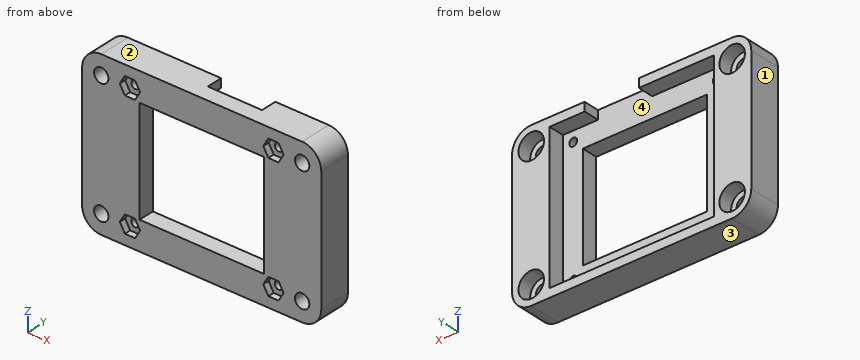
from build123d import *

# Parameters (mm, degrees)
SKETCH_1_W                   = 75
SKETCH_1_H                   = 51
EXTRUDE_1_DEPTH              = 10
SKETCH_2_W                   = 51.5
SKETCH_2_H                   = 45.5
CUT_EXTRUDE_1_DEPTH          = 5
SKETCH_3_R                   = 1.25
CUT_EXTRUDE_2_DEPTH          = 5
CUT_EXTRUDE_3_REACH          = 7
SKETCH_4_W                   = 39
SKETCH_4_H                   = 33
FILLET_1_R                   = 6
CUT_EXTRUDE_4_DEPTH          = 2
HOLE_WIZARD_M4_1_D           = 4.5
HOLE_WIZARD_M4_1_CBORE_D     = 8
HOLE_WIZARD_M4_1_CBORE_DEPTH = 4.4
SKETCH_7_W                   = 17
SKETCH_7_H                   = 2.75
CUT_EXTRUDE_5_DEPTH          = 5


with BuildPart() as part:
    # 草图1 → 凸台-拉伸1 (new body)
    with BuildSketch(Plane(origin=(0, 0, 0), x_dir=(1, 0, 0), z_dir=(0, 1, 0))):
        Rectangle(SKETCH_1_W, SKETCH_1_H)
    extrude(amount=EXTRUDE_1_DEPTH)

    # 草图2 → 切除-拉伸1 (cut)
    with BuildSketch(Plane(origin=(0, 10, 0), x_dir=(1, 0, 0), z_dir=(0, 1, 0))):
        Rectangle(SKETCH_2_W, SKETCH_2_H)
    extrude(amount=-CUT_EXTRUDE_1_DEPTH, mode=Mode.SUBTRACT)

    # 草图3 → 切除-拉伸2 (cut)
    with BuildSketch(Plane(origin=(0, 5, 0), x_dir=(1, 0, 0), z_dir=(0, 1, 0))):
        with Locations((-22.5, 19.5)):
            Circle(SKETCH_3_R)
        with Locations((-22.5, -19.5)):
            Circle(SKETCH_3_R)
        with Locations((22.5, -19.5)):
            Circle(SKETCH_3_R)
        with Locations((22.5, 19.5)):
            Circle(SKETCH_3_R)
    extrude(amount=-CUT_EXTRUDE_2_DEPTH, mode=Mode.SUBTRACT)

    # 草图4 → 切除-拉伸3 (cut, up to next)
    with BuildSketch(Plane(origin=(0, 5, 0), x_dir=(1, 0, 0), z_dir=(0, 1, 0)), mode=Mode.PRIVATE) as cut_extrude_3_sk1:
        Rectangle(SKETCH_4_W, SKETCH_4_H)
    cut_extrude_3_tool1 = extrude(cut_extrude_3_sk1.sketch, amount=-CUT_EXTRUDE_3_REACH, mode=Mode.PRIVATE) & part.part
    add(cut_extrude_3_tool1.solids().sort_by_distance((0, 5, 0))[0], mode=Mode.SUBTRACT)

    # 圆角1
    fillet_1_edges = [part.edges().sort_by_distance(p)[0] for p in [
        (37.5, 5, 25.5),
        (-37.5, 5, 25.5),
        (-37.5, 5, -25.5),
        (37.5, 5, -25.5),
    ]]
    fillet(fillet_1_edges, radius=FILLET_1_R)

    # 草图5 → 切除-拉伸4 (cut)
    with BuildSketch(Plane.XZ):
        Polygon((-19.324573519, 19.5), (-20.91228676, 22.25), (-24.08771324, 22.25), (-25.675426481, 19.5), (-24.08771324, 16.75), (-20.91228676, 16.75), align=None)
        Polygon((25.675426481, 19.5), (24.08771324, 22.25), (20.91228676, 22.25), (19.324573519, 19.5), (20.91228676, 16.75), (24.08771324, 16.75), align=None)
        Polygon((-19.324573519, -19.5), (-20.91228676, -16.75), (-24.08771324, -16.75), (-25.675426481, -19.5), (-24.08771324, -22.25), (-20.91228676, -22.25), align=None)
        Polygon((25.675426481, -19.5), (24.08771324, -16.75), (20.91228676, -16.75), (19.324573519, -19.5), (20.91228676, -22.25), (24.08771324, -22.25), align=None)
    extrude(amount=-CUT_EXTRUDE_4_DEPTH, mode=Mode.SUBTRACT)

    # M4 六角凹头螺钉的柱形沉头孔1 (through all)
    with Locations(Plane(origin=(31.5, 10, 19.5), x_dir=(0, 0, 1), z_dir=(0, 1, 0))):
        with Locations((0, 0), (-39, 0), (-39, -63), (0, -63)):
            CounterBoreHole(HOLE_WIZARD_M4_1_D / 2, HOLE_WIZARD_M4_1_CBORE_D / 2, HOLE_WIZARD_M4_1_CBORE_DEPTH)

    # 草图7 → 切除-拉伸5 (cut)
    with BuildSketch(Plane(origin=(0, 10, 0), x_dir=(1, 0, 0), z_dir=(0, 1, 0))):
        with Locations((6.25, -24.125)):
            Rectangle(SKETCH_7_W, SKETCH_7_H)
    extrude(amount=-CUT_EXTRUDE_5_DEPTH, mode=Mode.SUBTRACT)


solid = part.part
The model under review builds one solid part; all positions refer to its coordinate system, in mm. Face numbers are marked on the shaded views. Give positions to 0.01 mm unless a question says otherwise; leave off trailing zeros. Order: outer loops, then holes, each group sorted by start corner. A loop starts at its lowest first (then second) coordinate and runs counter-clockwise, first axis right, second up. Notation, with made-up numbers: M 74.5,37.5 L 125.5,37.5 A20 cw 125.5,62.5 Z; hole C 17,-27.75 d2. An arc over 180 degrees is marked long. One line per question, with ' | ' between items. Start each with the question number.
1) Consider section D-D, the plane x = -8. Give the boundary of the cut face in (y, z).
2) Consider section C-C, the plane y = 7. Give the boundary of the cut face in (x, z), then the cut area to 3 significant figures.
3) Clearance check with flat-ended pins moving along their axes: P1, Ø3, axis at x = 22.5, z = -19.5, coming from the +Y side; P2, Ø1.5, axis at x = -22.5, z = -19.5, coming from the +Y side; P3, Ø0.8, axis at y = 6.5, z = 24, coming from the +X side; P4, Ø1.5, axis at x = 4, y = 7, coming from the +Z side. State where each tip first meets the part, or that it passes through.
4) Mouldability with a two-part tool opening along Z and no side actions: class the marked faces 1, 2, 3 and 4 as pulls with the +Z half, pulls with the -Z half, needs draft (parallel to the pull), parting line crosses it, or undercut.
5) Consider section B-B, the plane z = 11.5. Give the boundary of the cut face in (x, y), then the cut area to 4 significant figures.
6) Wall thickness on L1, parallel to Z at x = -22.5, y = 3.45; L2, parallel to X at y = 2.7, z = 19.5; L3, parallel to X at y = 6.7, z = 19.5: over which ranges is each line inside the solid? List them lowest first. Write a range as from..to.
7) Consider section A-A, the plane x = 22.5. Give the boundary of the cut face in (y, z).
Found:
1) outline: M 0,-25.5 L 10,-25.5 L 10,-22.75 L 5,-22.75 L 5,-16.5 L 0,-16.5 Z; M 0,16.5 L 5,16.5 L 5,22.75 L 10,22.75 L 10,25.5 L 0,25.5 Z
2) outline: M -37.5,-19.5 A6 ccw -31.5,-25.5 L 31.5,-25.5 A6 ccw 37.5,-19.5 L 37.5,19.5 A6 ccw 31.5,25.5 L 14.75,25.5 L 14.75,22.75 L 25.75,22.75 L 25.75,-22.75 L -25.75,-22.75 L -25.75,22.75 L -2.25,22.75 L -2.25,25.5 L -31.5,25.5 A6 ccw -37.5,19.5 Z; hole C -31.5,-19.5 d8; hole C -31.5,19.5 d8; hole C 31.5,-19.5 d8; hole C 31.5,19.5 d8 | area: 1,200 mm²
3) P1: stops at y = 5 | P2: passes through | P3: stops at x = 35.88 | P4: stops at z = -22.75
4) face 1: needs draft | face 2: pulls with the +Z half | face 3: pulls with the -Z half | face 4: undercut
5) outline: M -37.5,0 L -19.5,0 L -19.5,5 L -25.75,5 L -25.75,10 L -37.5,10 Z; M 19.5,0 L 37.5,0 L 37.5,10 L 25.75,10 L 25.75,5 L 19.5,5 Z | area: 297.5 mm²
6) L1: z = -25.5..-20.75, -18.25..18.25, 20.75..25.5 | L2: x = -37.5..-33.75, -29.25..-23.75, -21.25..21.25, 23.75..29.25, 33.75..37.5 | L3: x = -37.5..-35.5, -27.5..-25.75, 25.75..27.5, 35.5..37.5
7) outline: M 0,-25.5 L 10,-25.5 L 10,-22.75 L 5,-22.75 L 5,-20.75 L 2,-20.75 L 2,-22.25 L 0,-22.25 Z; M 0,-16.75 L 2,-16.75 L 2,-18.25 L 5,-18.25 L 5,18.25 L 2,18.25 L 2,16.75 L 0,16.75 Z; M 0,22.25 L 2,22.25 L 2,20.75 L 5,20.75 L 5,22.75 L 10,22.75 L 10,25.5 L 0,25.5 Z
